Autodesk Inventor part; units mm, degrees
ref_plane "YZ Plane" through (0, 0, 0) normal (1, 0, 0) x (0, 1, 0)
ref_plane "XZ Plane" through (0, 0, 0) normal (0, 1, 0) x (-1, 0, 0)
ref_plane "XY Plane" through (0, 0, 0) normal (0, 0, 1) x (1, 0, 0)
sketch "Sketch1" plane through (0, 0, 0) normal (0, 1, 0) x (-1, 0, 0)
  line L0 (12.113, -8) -> (-12.113, -8)
  line L1 (-12.113, 8) -> (12.113, 8)
  arc A0 (12.113, -8) -> (12.113, 8) centre (12.113, 0) ccw
  arc A1 (-12.113, 8) -> (-12.113, -8) centre (-12.113, 0) ccw
  point P0 (0, 0)
  dimension "d0" = 16
  dimension "d2" = 8
  dimension "d4" = 24.226
  dimension "d5" = 12.113
extrude "Extrusion1" add sketch "Sketch1" along normal blind 7.5
sketch "Sketch2" plane through (0, 7.5, 0) normal (0, 1, 0) x (1, 0, 0)
  arc A0 (-12.113, 8) -> (-12.113, -8) centre (-12.113, 0) ccw
  arc A1 (12.113, -8) -> (12.113, 8) centre (12.113, 0) ccw
  point P0 (0, 0)
  point P1 (-12.113, 0)
  point P2 (12.113, 0)
  dimension "d8" = 0
  dimension "d9" = 0
  dimension "d11" = 0
  dimension "d12" = 0
hole "Hole1" at (12.113, 7.5, 0) at (-12.113, 7.5, 0) direction (0, -1, 0) diameter 8 end through all
sketch "Sketch3" plane through (-12.113, 0, 8) normal (0, 0, 1) x (1, 0, 0)
  line L0 (24.226, 7.5) -> (0, 7.5)
  line L1 (24.226, 0) -> (0, 0)
  line L2 (4.613, 7.5) -> (19.613, 7.5)
  line L3 (19.613, 7.5) -> (19.613, 0)
  line L4 (19.613, 0) -> (4.613, 0)
  line L5 (4.613, 0) -> (4.613, 7.5)
  point P0 (12.113, 0)
  point P1 (4.613, 0)
  dimension "d20" = 15
  dimension "d21" = 7.5
extrude "Extrusion2" add sketch "Sketch3" along normal blind 30
fillet "Fillet1" radius 2 2 edges at (-7.5, 3.75, 8) (7.5, 3.75, 8)
properties part number "holder3_puller"
Design review of the part built by this model. Coordinates are the model's own, in mm. A direction names the side the tool comes from. Coordinates: 2 decimals unless noted, no trailing zeros. Order: outer loops, then holes, each group sorted by start corner. A loop starts at its lowest first (then second) coordinate and runs counter-clockwise, first axis right, second up. Notation, with made-up numbers: (63.25, -33.5) -> (98.25, -33.5) arc R12 cw to (98.25, -25.5) -> close; hole circle Ø4 at (82, 29.5). An arc over 180 degrees is marked (long way). One line per item, written item: value.
1) To check wall thickness, follow probe 1 along X at (y, z) = (4.5, 0); probe 2 along Z at (x, y) = (-12, 6.5); probe 3 along X at (y, z) = (7, 10). State the ranges of each line that lie inside material, in increasing order. Write a range as [from, to].
Output values:
probe 1: x = [-20.11, -16.11], [-8.11, 8.11], [16.11, 20.11]
probe 2: z = [-8, -4], [4, 8]
probe 3: x = [-7.5, 7.5]
2) We need section B-B, the plane y = 4.5. Give the boundary of the cut face in (x, z).
Output values:
outline: (-12.11, -8) -> (12.11, -8) arc R8 ccw to (12.11, 8) -> (9.5, 8) arc R2 cw to (7.5, 10) -> (7.5, 38) -> (-7.5, 38) -> (-7.5, 10) arc R2 cw to (-9.5, 8) -> (-12.11, 8) arc R8 ccw to start; hole circle Ø8 at (-12.11, 0); hole circle Ø8 at (12.11, 0)
3) We need section C-C, the plane x = 11. Give the boundary of the cut face in (y, z), then the cut area to 3 significant figures.
Output values:
outline: (0, -8) -> (7.5, -8) -> (7.5, -3.84) -> (0, -3.84) -> close; (0, 3.84) -> (7.5, 3.84) -> (7.5, 8) -> (0, 8) -> close
area: 62.4 mm2
4) Draft analysis for pull direction Z (two halves, no side actions). For faces 4 (the face through (8.07, 3.7, 8.6)), 5 (the face through (-8.21, 3.7, -0.87)), 6 (the face through (0, 7.5, 10)), 7 (the face through (20.11, 3.7, -0.18)), state which applies: +Z half, -Z half, draft (parallel to the pull), parting line (faces both ways), or undercut.
Output values:
face 4: +Z half
face 5: undercut
face 6: draft
face 7: parting line
5) We need section D-D, the plane z = 32.5. Give the boundary of the cut face in (x, y).
Output values:
outline: (-7.5, 0) -> (7.5, 0) -> (7.5, 7.5) -> (-7.5, 7.5) -> close
6) Clearance check with flat-ended pins moving along their axes: P1, Ø6.5, axis at x = 12.113, z = 0, coming from the +Y side; P2, Ø5, axis at x = 2, z = 21.5, coming from the -Y side; P3, Ø1, axis at y = 6, z = 17.5, coming from the -X side; P4, Ø3, axis at x = 10.5, y = 2, coming from the +Z side. State where each tip first meets the part, or that it passes through.
Output values:
P1: passes through
P2: stops at y = 0
P3: stops at x = -7.5
P4: stops at z = 8.06
7) We need section A-A, the plane z = 0. Give the boundary of the cut face in (x, y).
Output values:
outline: (-20.11, 0) -> (-16.11, 0) -> (-16.11, 7.5) -> (-20.11, 7.5) -> close; (-8.11, 0) -> (8.11, 0) -> (8.11, 7.5) -> (-8.11, 7.5) -> close; (16.11, 0) -> (20.11, 0) -> (20.11, 7.5) -> (16.11, 7.5) -> close
8) Machinability: for faces 1 (the face through (11, 4, 8)), 2 (the face through (-11, 4, 8)), 3 (the face through (-20.11, 3.7, 0.18)), which of the approach directions +Z, -Z, +X, -X, +Y, -Y give a long, thin tool a straight path to every point of the face, cutting with its end or side? Answer none if there is none.
Output values:
face 1: +Z, +X, +Y, -Y
face 2: +Z, -X, +Y, -Y
face 3: -X, +Y, -Y
